Part model, mm, in its own coordinate system. A direction names the side the tool comes from. Round coordinates to 2 decimals unless told otherwise and drop trailing zeros. Write each loop counter-clockwise with the first axis right and the second up, starting at its lowest first coordinate (ties: lowest second). Pieces come first, ordered by that corner, then holes.
```python
from build123d import *

# Parameters (mm, degrees)
EXTRUDE_THIN1_DEPTH = 563.5625
FILLET1_R           = 1.016


with BuildPart() as part:
    # Sketch1 → Extrude-Thin1 (new body)
    with BuildSketch(Plane.XY):
        with BuildLine():
            Line((0, 0), (-9.525, 0))
            Line((-9.525, 0), (-9.525, 43.65625))
            Line((-9.525, 43.65625), (-7.9375, 43.65625))
            ThreePointArc((-7.9375, 43.65625), (-6.894744616, 50.081998205), (-3.8735, 55.84825))
            ThreePointArc((-3.8735, 55.84825), (-2.455890737, 56.291077789), (-1.5875, 55.08625))
            Line((-1.5875, 55.08625), (-1.5875, 53.18125))
            Line((-1.5875, 53.18125), (0, 53.18125))
            Line((0, 53.18125), (0, 52.16525))
            Line((0, 52.16525), (-2.6035, 52.16525))
            Line((-2.6035, 52.16525), (-2.6035, 55.08625))
            ThreePointArc((-2.6035, 55.08625), (-2.777178147, 55.327215558), (-3.0607, 55.23865))
            ThreePointArc((-3.0607, 55.23865), (-6.085235087, 49.276497038), (-6.894744616, 42.64025))
            Line((-6.894744616, 42.64025), (-8.509, 42.64025))
            Line((-8.509, 42.64025), (-8.509, 1.016))
            Line((-8.509, 1.016), (0, 1.016))
            Line((0, 1.016), (0, 0))
        make_face()
    extrude(amount=-EXTRUDE_THIN1_DEPTH)

    # Fillet1
    fillet1_edges = [part.edges().sort_by_distance(p)[0] for p in [
        (-2.6035, 52.16525, -281.78125),
        (-6.894744616, 42.64025, -281.78125),
        (-9.525, 0, -281.78125),
        (-9.525, 43.65625, -281.78125),
    ]]
    fillet(fillet1_edges, radius=FILLET1_R)


solid = part.part
```
Q1. Wall check: L1, parallel to Y at x = -8.25, z = -221; L2, parallel to Y at x = -1, z = -124; L3, parallel to X at y = 6, z = -442 (3 decimals). Give the ranges that are in metal, low to high.
Values follow:
L1: y = 0 to 1.02, 42.64 to 43.66
L2: y = 0 to 1.02, 52.17 to 53.18
L3: x = -9.525 to -8.509
Q2. Cut at B-B on y = 15. Write the cut outline in (x, z) (1 decimal).
Values follow:
outline: (-9.5, -563.6) - (-8.5, -563.6) - (-8.5, 0) - (-9.5, 0) - close
Q3. Which spindle directions (+Z, -Z, +X, -X, +Y, -Y) get a long thin tool onto all of the face, cutting with end or side? Do faces 1 (the flat face through (-4, 0, -278)), 2 (the flat face through (-8.509, 22, -278)), 3 (the cylindrical face through (-5.903, 49.843, -277.836)). Say none if no direction does.
Values follow:
face 1: +Z, -Z, +X, -X, -Y
face 2: +Z, -Z, +X
face 3: +Z, -Z
Q4. Cut at A-A on z = -292. Write the cut outline in (x, y) (1 decimal), plus the area to 3 significant figures.
Values follow:
outline: (-9.5, 1) arc R1 ccw to (-8.5, 0) - (0, 0) - (0, 1) - (-8.5, 1) - (-8.5, 42.6) - (-7.9, 42.6) arc R1 ccw to (-6.9, 43.7) arc R19.3 cw to (-3.1, 55.2) arc R0.3 cw to (-2.6, 55.1) - (-2.6, 53.2) arc R1 ccw to (-1.6, 52.2) - (0, 52.2) - (0, 53.2) - (-1.6, 53.2) - (-1.6, 55.1) arc R1.3 ccw to (-3.9, 55.8) arc R20.3 ccw to (-7.9, 43.7) - (-8.5, 43.7) arc R1 ccw to (-9.5, 42.6) - close
area: 73.2 mm2
Q5. Drop flat-ended pins along their axis: pin 1 (1.7 mm diameter, centred on x = -0.5, z = -248.5, fed in from +Y); pin 2 (0.6 mm diameter, centred on y = 54.5, z = -181.5, fed in from +X); pin 3 (2.5 mm diameter, centred on x = -6, z = -390, fed in from +Y). Give the stop position or say it passes through.
Values follow:
pin 1: stops at y = 53.18
pin 2: stops at x = -1.59
pin 3: stops at y = 54.58
Q6. Mould opens along Y. For faces 4 (the flat face through (-9.525, 22, -278)), 5 (the cylindrical face through (-6.92, 50, -277.84)), 6 (the flat face through (-4, 1.016, -278)) say: +Y half, -Y half, draft (parallel to the pull), parting line (faces both ways), or undercut.
Values follow:
face 4: draft
face 5: +Y half
face 6: undercut
